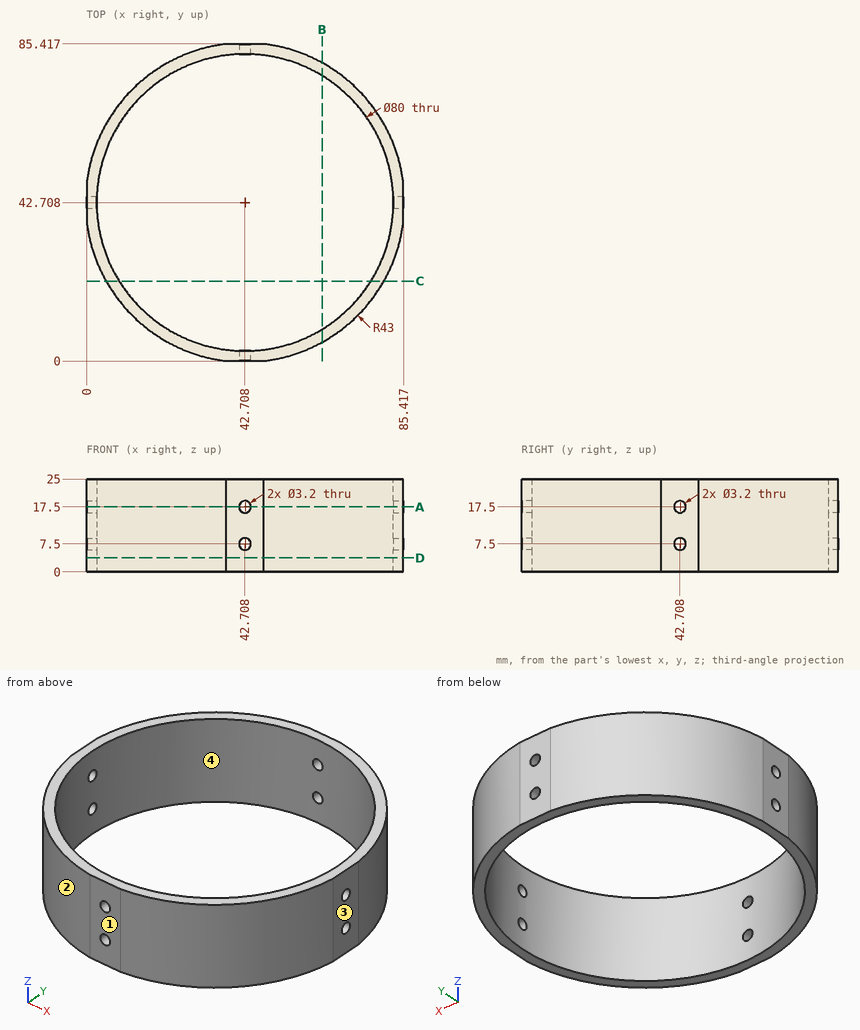
Study the drawing (mm; zero at the part's minimum x, y, z) and answer. Round coordinates to 2 decimals unless told otherwise and drop trailing zeros. Write each loop counter-clockwise with the first axis right and the second up, starting at its lowest first coordinate (ties: lowest second). Pieces come first, ordered by that corner, then holes.
1) Given pin 1 Ø1.5 at (y, z) = (74, 11) entering from -X; pin 2 Ø12 at (x, z) = (68.5, 18) entering from -Y; pin 3 Ø12 at (x, z) = (23, 17) entering from +Y (1 decimal), each flat-ended and moving along its own axis, determine where each tip first touches the part or whether it passes through.
2) A cutting plane is placed at B-B (x = 63.5). Give the vertices of the cut face in (y, z).
3) The mould has two halves that part along X. Classify the marked faces 1, 2, 3 and 4: pulls with the +X half, pulls with the -X half, needs draft (parallel to the pull), parting line crosses it, or undercut.
4) A cutting plane is placed at D-D (z = 3.75). Give the vertices of the cut face in (x, y).
5) A cutting plane is placed at C-C (y = 21.5). Give the vertices of the cut face in (x, z) (1 decimal).
6) Straight lines are drawn through the part: line 1 (Y direction, x = 43.5, z = 19.25); line 2 (X direction, y = 15, z = 11.25) (1 decimal); line 3 (X direction, y = 16.5, z = 17.5) (1 decimal). For each, find the intervals that lie inside material, in ascending order.
7) A cutting plane is placed at A-A (z = 17.5). Give the vertices of the cut face in (x, y).
Completed:
1. pin 1: stops at x = 12.44
1. pin 2: stops at y = 4.53
1. pin 3: stops at y = 83.5
2. outline: (5.07, 0) - (8.54, 0) - (8.54, 25) - (5.07, 25) - close; (76.88, 0) - (80.35, 0) - (80.35, 25) - (76.88, 25) - close
3. face 1: needs draft
3. face 2: pulls with the -X half
3. face 3: pulls with the +X half
3. face 4: undercut
4. outline: (0, 37.71) arc R43 ccw to (37.71, 0) - (47.71, 0) arc R43 ccw to (85.42, 37.71) - (85.42, 47.71) arc R43 ccw to (47.71, 85.42) - (37.71, 85.42) arc R43 ccw to (0, 47.71) - close; hole circle Ø80 at (42.71, 42.71)
5. outline: (5.3, 0) - (8.8, 0) - (8.8, 25) - (5.3, 25) - close; (76.6, 0) - (80.1, 0) - (80.1, 25) - (76.6, 25) - close
6. line 1: y = 0 to 2.72, 82.7 to 85.42
6. line 2: x = 9.8 to 13.9, 71.6 to 75.6
6. line 3: x = 8.6 to 12.5, 72.9 to 76.8
7. outline: (0, 37.71) arc R43 ccw to (37.71, 0) - (41.11, 0) - (41.11, 2.74) arc R40 cw to (2.74, 41.11) - (0, 41.11) - close; (0, 44.31) - (2.74, 44.31) arc R40 cw to (41.11, 82.68) - (41.11, 85.42) - (37.71, 85.42) arc R43 ccw to (0, 47.71) - close; (44.31, 0) - (47.71, 0) arc R43 ccw to (85.42, 37.71) - (85.42, 41.11) - (82.68, 41.11) arc R40 cw to (44.31, 2.74) - close; (44.31, 82.68) arc R40 cw to (82.68, 44.31) - (85.42, 44.31) - (85.42, 47.71) arc R43 ccw to (47.71, 85.42) - (44.31, 85.42) - close
